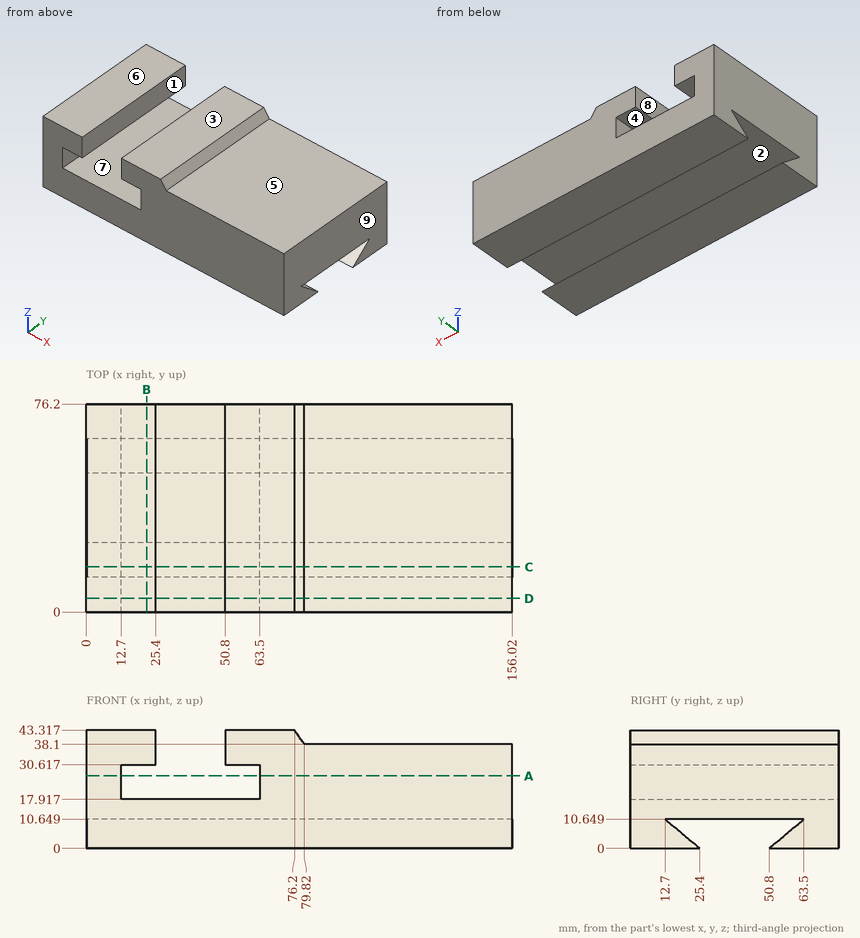
Geometry check sheet. Reference: drawing and pictorial views, mm from the part's lowest x, y, z. A direction names the side the tool comes from. Round coordinates to 2 decimals unless told otherwise and drop trailing zeros. Order: outer loops, then holes, each group sorted by start corner. A loop starts at its lowest first (then second) coordinate and runs counter-clockwise, first axis right, second up. Notation, with made-up numbers: (-14.75, -3.5) - (31.25, -3.5) arc R20 cw to (31.25, 26.5) - close; hole circle Ø3 at (74, -39.75). An arc over 180 degrees is marked (long way). Use a Markdown table: item, result. Add a question column.
1) Section check D-D (y = 5). Record the cut outline in (x, z).
2) Set-up check for the marked faces 1, 2, 3, 4 and 5: record each of +Z, -Z, +X, -X, +Y, -Y from which the full face is reachable in a straight line by a thin tool's end or side.
3) Section check B-B (x = 22). Record the cut outline in (y, z), then the cut area to 3 significant figures.
4) Gauge pin test, flat ends, axial feed: P1, Ø23, axis at x = 107, y = 37, coming from the +Z side; P2, Ø15, axis at x = 58.5, y = 35.5, coming from the -Z side. Record the tip position at first contact, or that the pin passes through.
5) Section check A-A (z = 26.5). Record the cut outline in (x, y).
6) Thickness scan on line 1 along X through (y, z) = (38, 27); line 2 along Z through (x, y) = (146, 27); line 3 along Z through (x, y) = (24, 58.5). Record the ranges inside material, lowest first.
7) Section check C-C (y = 16.5). Record the cut outline in (x, z).
8) Mould release check, pull along X, two halves, no side actions. Record for the marked faces 6, 7, 8 and 9: released by +X, released by -X, zero draft, split by the parting line, or undercut.
Established:
| question | item | result |
|---|---|---|
| 1 | outline | (0, 0) - (156.02, 0) - (156.02, 38.1) - (79.82, 38.1) - (76.2, 43.32) - (50.8, 43.32) - (50.8, 30.62) - (63.5, 30.62) - (63.5, 17.92) - (12.7, 17.92) - (12.7, 30.62) - (25.4, 30.62) - (25.4, 43.32) - (0, 43.32) - close |
| 2 | face 1 | +Z, +Y, -Y |
| 2 | face 2 | +X, -X |
| 2 | face 3 | +Z, +X, -X, +Y, -Y |
| 2 | face 4 | +Y, -Y |
| 2 | face 5 | +Z, +X, +Y, -Y |
| 3 | outline | (0, 0) - (25.4, 0) - (12.7, 10.65) - (63.5, 10.65) - (50.8, 0) - (76.2, 0) - (76.2, 17.92) - (0, 17.92) - close; (0, 30.62) - (76.2, 30.62) - (76.2, 43.32) - (0, 43.32) - close |
| 3 | area | 1,930 mm2 |
| 4 | P1 | z = 38.1 |
| 4 | P2 | z = 10.65 |
| 5 | outline | (0, 0) - (12.7, 0) - (12.7, 76.2) - (0, 76.2) - close; (63.5, 0) - (156.02, 0) - (156.02, 76.2) - (63.5, 76.2) - close |
| 6 | line 1 | 0 to 12.7, 63.5 to 156.02 |
| 6 | line 2 | 10.65 to 38.1 |
| 6 | line 3 | 0 to 6.46, 10.65 to 17.92, 30.62 to 43.32 |
| 7 | outline | (0, 0) - (156.02, 0) - (156.02, 7.46) - (0, 7.46) - close; (0, 10.65) - (156.02, 10.65) - (156.02, 38.1) - (79.82, 38.1) - (76.2, 43.32) - (50.8, 43.32) - (50.8, 30.62) - (63.5, 30.62) - (63.5, 17.92) - (12.7, 17.92) - (12.7, 30.62) - (25.4, 30.62) - (25.4, 43.32) - (0, 43.32) - close |
| 8 | face 6 | zero draft |
| 8 | face 7 | undercut |
| 8 | face 8 | undercut |
| 8 | face 9 | released by +X |
